Check sheet for the modelled part. Datum: model origin and axes. Units: mm. A direction names the side the tool comes from. Give positions to 0.01 mm unless a question says otherwise; leave off trailing zeros. Write each loop counter-clockwise with the first axis right and the second up, starting at its lowest first coordinate (ties: lowest second). Pieces come first, ordered by that corner, then holes. Notation, with made-up numbers: (38, 43.25) -> (91, 43.25) arc R17 cw to (91, 70.25) -> close; hole circle Ø2 at (37, 56.25). An arc over 180 degrees is marked (long way). Return JSON: item names as keys, results as strings.
from build123d import *

# Parameters (mm, degrees)
SKETCH1_W           = 5
SKETCH1_H           = 5
BOSS_EXTRUDE1_DEPTH = 2
SKETCH2_W           = 3.2
SKETCH2_H           = 3
BOSS_EXTRUDE2_DEPTH = 5
SKETCH3_W           = 3.2
SKETCH3_H           = 3.6
BOSS_EXTRUDE3_DEPTH = 3
CUT_EXTRUDE1_DEPTH  = 12.093241186
SKETCH6_W           = 5
SKETCH6_H           = 2
CUT_EXTRUDE2_DEPTH  = 12.456439237
SKETCH7_W           = 18
SKETCH7_H           = 4
BOSS_EXTRUDE5_DEPTH = 13
SKETCH8_W           = 18
SKETCH8_H           = 6
BOSS_EXTRUDE6_DEPTH = 4
SKETCH9_W           = 1.5
SKETCH9_H           = 2
CUT_EXTRUDE4_DEPTH  = 22.800229357
SKETCH10_W          = 1
SKETCH10_H          = 9
CUT_EXTRUDE5_DEPTH  = 22.800229357
CUT_EXTRUDE6_DEPTH  = 22.800229357
BOSS_EXTRUDE7_DEPTH = 0.6
SKETCH13_W          = 3.9
SKETCH13_H          = 5.5
BOSS_EXTRUDE8_DEPTH = 3.2
CHAMFER2_SIZE       = 2.5
CHAMFER2_SIZE2      = 4.330127019
SKETCH14_W          = 8
SKETCH14_H          = 1.75299242
CUT_EXTRUDE7_DEPTH  = 22.800229515
SKETCH16_W          = 18
SKETCH16_H          = 4.24700758
BOSS_EXTRUDE9_DEPTH = 0.6
CHAMFER4_SIZE       = 2.2
CHAMFER4_SIZE2      = 3.141925615
CHAMFER5_SIZE       = 0.5
FILLET1_R           = 1


with BuildPart() as part:
    # Sketch1 → Boss-Extrude1 (new body)
    with BuildSketch(Plane(origin=(0, 0, 0), x_dir=(1, 0, 0), z_dir=(0, 1, 0))):
        Rectangle(SKETCH1_W, SKETCH1_H)
    extrude(amount=BOSS_EXTRUDE1_DEPTH)

    # Sketch2 → Boss-Extrude2 (add)
    with BuildSketch(Plane(origin=(0, 2, 0), x_dir=(1, 0, 0), z_dir=(0, 1, 0))):
        with Locations((0, 1)):
            Rectangle(SKETCH2_W, SKETCH2_H)
    extrude(amount=BOSS_EXTRUDE2_DEPTH)

    # Sketch3 → Boss-Extrude3 (add)
    with BuildSketch(Plane(origin=(0, 7, 0), x_dir=(1, 0, 0), z_dir=(0, 1, 0))):
        with Locations((0, 0.7)):
            Rectangle(SKETCH3_W, SKETCH3_H)
    extrude(amount=BOSS_EXTRUDE3_DEPTH)

    # Sketch4 → Cut-Extrude1 (cut, through all)
    with BuildSketch(Plane(origin=(1.6, 0, 0), x_dir=(0, 0, -1), z_dir=(1, 0, 0))):
        Polygon((-1.1, 7), (0.75, 10), (-1.1, 10), align=None)
    extrude(amount=-CUT_EXTRUDE1_DEPTH, mode=Mode.SUBTRACT)

    # Sketch6 → Cut-Extrude2 (cut, through all)
    with BuildSketch(Plane.XY.offset(2.5)):
        with Locations((0, 1)):
            Rectangle(SKETCH6_W, SKETCH6_H)
    extrude(amount=-CUT_EXTRUDE2_DEPTH, mode=Mode.SUBTRACT)

    # Sketch7 → Boss-Extrude5 (add)
    with BuildSketch(Plane.XZ.offset(-2)):
        with Locations((0, -0.5)):
            Rectangle(SKETCH7_W, SKETCH7_H)
    extrude(amount=BOSS_EXTRUDE5_DEPTH)

    # Sketch8 → Boss-Extrude6 (add)
    with BuildSketch(Plane.XY.offset(1.5)):
        with Locations((0, -8)):
            Rectangle(SKETCH8_W, SKETCH8_H)
    extrude(amount=BOSS_EXTRUDE6_DEPTH)

    # Sketch9 → Cut-Extrude4 (cut, through all)
    with BuildSketch(Plane(origin=(9, 0, 0), x_dir=(0, 0, -1), z_dir=(1, 0, 0))):
        with Locations((-2.25, -6)):
            Rectangle(SKETCH9_W, SKETCH9_H)
    extrude(amount=-CUT_EXTRUDE4_DEPTH, mode=Mode.SUBTRACT)

    # Sketch10 → Cut-Extrude5 (cut, through all)
    with BuildSketch(Plane(origin=(9, 0, 0), x_dir=(0, 0, -1), z_dir=(1, 0, 0))):
        with Locations((-1, -2.5)):
            Rectangle(SKETCH10_W, SKETCH10_H)
    extrude(amount=-CUT_EXTRUDE5_DEPTH, mode=Mode.SUBTRACT)

    # Sketch11 → Cut-Extrude6 (cut, through all)
    with BuildSketch(Plane(origin=(9, 0, 0), x_dir=(0, 0, -1), z_dir=(1, 0, 0))):
        with BuildLine():
            Line((-0.5, 0.906362555), (-0.5, -7))
            add(Edge.make_bspline(
                [(-0.5, 0.906362555), (4.232995097, -2.809658902), (-0.5, -7)],
                knots=[0, 0, 0, 1, 1, 1], degree=2))
        make_face()
    extrude(amount=-CUT_EXTRUDE6_DEPTH, mode=Mode.SUBTRACT)

    # Sketch12 → Boss-Extrude7 (add)
    with BuildSketch(Plane.XY.offset(0.5)):
        Polygon((-9, 2), (-9, 0.906362555), (9, 0.906362555), (9, 2), (1.6, 2), (1.6, 7), (-1.6, 7), (-1.6, 2), align=None)
    extrude(amount=BOSS_EXTRUDE7_DEPTH)

    # Sketch13 → Boss-Extrude8 (add)
    with BuildSketch(Plane.ZY.offset(1.6)):
        with Locations((-0.55, 7.25)):
            Rectangle(SKETCH13_W, SKETCH13_H)
    extrude(amount=-BOSS_EXTRUDE8_DEPTH)

    # Chamfer2
    chamfer2_edges = [part.edges().sort_by_distance(p)[0] for p in [
        (0, 10, 1.4),
    ]]
    chamfer2_side = [part.faces().sort_by_distance(p)[0] for p in [
        (0, 10, -0.55),
    ]]
    chamfer(chamfer2_edges, length=CHAMFER2_SIZE, length2=CHAMFER2_SIZE2, reference=chamfer2_side[0])

    # Sketch14 → Cut-Extrude7 (cut, through all)
    with BuildSketch(Plane(origin=(9, 0, 0), x_dir=(0, 0, -1), z_dir=(1, 0, 0))):
        with Locations((-1.5, -10.12350379)):
            Rectangle(SKETCH14_W, SKETCH14_H)
    extrude(amount=-CUT_EXTRUDE7_DEPTH, mode=Mode.SUBTRACT)

    # Sketch16 → Boss-Extrude9 (add)
    with BuildSketch(Plane.XY.offset(5.5)):
        with Locations((0, -7.12350379)):
            Rectangle(SKETCH16_W, SKETCH16_H)
    extrude(amount=BOSS_EXTRUDE9_DEPTH)

    # Chamfer4
    chamfer4_edges = [part.edges().sort_by_distance(p)[0] for p in [
        (0, -9.24700758, 6.1),
    ]]
    chamfer4_side = [part.faces().sort_by_distance(p)[0] for p in [
        (0, -9.24700758, 1.8),
    ]]
    chamfer(chamfer4_edges, length=CHAMFER4_SIZE, length2=CHAMFER4_SIZE2, reference=chamfer4_side[0])

    # Chamfer5
    chamfer5_edges = [part.edges().sort_by_distance(p)[0] for p in [
        (0, -5, 3),
        (0, -5, 6.1),
    ]]
    chamfer(chamfer5_edges, length=CHAMFER5_SIZE)

    # Fillet1
    fillet1_edges = [part.edges().sort_by_distance(p)[0] for p in [
        (0, -9.24700758, -2.5),
    ]]
    fillet(fillet1_edges, radius=FILLET1_R)


solid = part.part
(1) Set-up check for faces 1 (the flat face through (0, 5, 1.4)), 2 (the flat face through (0, -7, 2)), 3 (the flat face through (-1.6, 6, -1)), 4 (the flat face through (1.6, 6, -1)): record each of +Z, -Z, +X, -X, +Y, -Y from which the full face is reachable in a straight line by a thin tool's end or side.
Reply:
{"face 1": "+Z, +X, -X, +Y", "face 2": "+X, -X", "face 3": "+Z, -Z, -X, +Y", "face 4": "+Z, -Z, +X, +Y"}
(2) Depth check by flat-ended pin: pin 1 Ø3 at (x, z) = (4.5, -1) entering from +Y; pin 2 Ø3 at (x, z) = (0, 2) entering from +Y; pin 3 Ø2 at (y, z) = (6, -1.5) entering from +X; pin 4 Ø2 at (y, z) = (4.5, 4) entering from -X. Enter the tip coordinate at first touch or a pass-through.
Reply:
{"pin 1": "y = 2", "pin 2": "y = 7.23", "pin 3": "x = 1.6", "pin 4": "through"}
(3) Release check for a two-part mould opening along Y. For faces 5 (the flat face through (-9, -6, -1)), 6 (the flat face through (-0.02, 7.8, 0.17)), 7 (the flat face through (0, 2, 1.1)), 8 (the flat face through (0, -9.247, 1)) record: pulls with the +Y half, pulls with the -Y half, needs draft (parallel to the pull), parting line crosses it, or undercut.
Reply:
{"face 5": "needs draft", "face 6": "pulls with the +Y half", "face 7": "undercut", "face 8": "pulls with the -Y half"}
(4) Cross-section at B-B on y = 1.25. Enter the section's corners in (x, z).
Reply:
{"outline": "(-9, -2.5) -> (9, -2.5) -> (9, 1.1) -> (-9, 1.1) -> close"}
(5) Cross-section at A-A on z = 2.25. Enter the section's corners in (x, y).
Reply:
{"outline": "(-9, -9.25) -> (9, -9.25) -> (9, -7) -> (-9, -7) -> close"}
(6) Thickness scan on L1, parallel to Y at x = 4.25, z = 1; L2, parallel to Z at x = -8, y = 1.25; L3, parallel to Y at x = -0.5, z = 1.25. Record the ranges inside material, lowest first.
Reply:
{"L1": "-9.25 to -7, 0.91 to 2", "L2": "-2.5 to 1.1", "L3": "-9.25 to -7, 4.5 to 5.93"}
